```python
from build123d import *

# Parameters (mm, degrees)
SKETCH1_W           = 96
SKETCH1_H           = 68
BOSS_EXTRUDE1_DEPTH = 5
SKETCH2_R           = 1.65
SKETCH2_R_2         = 1.6
SKETCH2_R_3         = 7.5
CUT_EXTRUDE1_DEPTH  = 60.033888573


with BuildPart() as part:
    # Sketch1 → Boss-Extrude1 (new body)
    with BuildSketch(Plane(origin=(0, 0, 0), x_dir=(1, 0, 0), z_dir=(0, 1, 0))):
        Rectangle(SKETCH1_W, SKETCH1_H)
    extrude(amount=BOSS_EXTRUDE1_DEPTH)

    # Sketch2 → Cut-Extrude1 (cut, through all)
    with BuildSketch(Plane(origin=(0, 5, 0), x_dir=(1, 0, 0), z_dir=(0, 1, 0))):
        with Locations(Location((-43, 14, 0), (0, 0, 270))):
            Circle(SKETCH2_R)
        with Locations(Location((43, 14, 0), (0, 0, 270))):
            Circle(SKETCH2_R)
        with Locations(Location((43, -14, 0), (0, 0, 270))):
            Circle(SKETCH2_R)
        with Locations(Location((-43, -14, 0), (0, 0, 270))):
            Circle(SKETCH2_R)
        with Locations(Location((-11, 8, 0), (0, 0, 270))):
            Circle(SKETCH2_R_2)
        with Locations(Location((33, 8, 0), (0, 0, 270))):
            Circle(SKETCH2_R_2)
        with Locations(Location((33, -17, 0), (0, 0, 270))):
            Circle(SKETCH2_R_2)
        with Locations(Location((-11, -17, 0), (0, 0, 270))):
            Circle(SKETCH2_R_2)
        with Locations(Location((11, -3, 0), (0, 0, 270))):
            Circle(SKETCH2_R_3)
    extrude(amount=-CUT_EXTRUDE1_DEPTH, mode=Mode.SUBTRACT)


solid = part.part
```
The listing builds one solid part. Answer for the finished solid, in the listing's coordinates (mm). Give positions to 0.01 mm unless a question says otherwise; leave off trailing zeros. Order: outer loops, then holes, each group sorted by start corner. A loop starts at its lowest first (then second) coordinate and runs counter-clockwise, first axis right, second up. Notation, with made-up numbers: (29, 49.25) -> (65, 49.25) arc R33 cw to (65, 85.25) -> close; hole circle Ø7 at (81, 5). An arc over 180 degrees is marked (long way). Answer as a JSON object with one key per item and string values. Group by question number.
Item 1: The part is cut by section D-D on y = 3.5. Give the number of separate pieces and of enclosed holes in the cut face, and give its area (3 significant figures).
Item 2: The part is cut by section B-B on z = -14. Write down the section's boundary in (x, y).
Item 3: Consider L1, parallel to X at y = 3.5, z = -8; L2, parallel to X at y = 2, z = 14; L3, parallel to Z at x = -42, y = 2.5. Determine where each line is inside the solid, lowest interval first. Write a range as from..to.
Item 4: The part is cut by section C-C on x = 11. Write down the section's boundary in (y, z), and give its area (3 significant figures).
Item 5: The part is cut by section A-A on x = 43. Write down the section's boundary in (y, z), and give its area (3 significant figures).
Item 6: Determine the mould class of faces 1 (the cylindrical face through (32.03, 2.54, 15.73)), 2 (the flat face through (-1, 5, 0)), 3 (the flat face through (-1, 2, -34)) for opening direction Z: pulls with the +Z half, pulls with the -Z half, needs draft (parallel to the pull), parting line crosses it, or undercut.
Result set:
{
 "1": {"separate pieces": "1", "enclosed holes": "9", "area": "6,280 mm²"},
 "2": {"outline": "(-48, 0) -> (-44.65, 0) -> (-44.65, 5) -> (-48, 5) -> close; (-41.35, 0) -> (41.35, 0) -> (41.35, 5) -> (-41.35, 5) -> close; (44.65, 0) -> (48, 0) -> (48, 5) -> (44.65, 5) -> close"},
 "3": {"L1": "-48..-12.6, -9.4..31.4, 34.6..48", "L2": "-48..-44.65, -41.35..41.35, 44.65..48", "L3": "-34..-15.31, -12.69..12.69, 15.31..34"},
 "4": {"outline": "(0, -34) -> (5, -34) -> (5, -4.5) -> (0, -4.5) -> close; (0, 10.5) -> (5, 10.5) -> (5, 34) -> (0, 34) -> close", "area": "265 mm²"},
 "5": {"outline": "(0, -34) -> (5, -34) -> (5, -15.65) -> (0, -15.65) -> close; (0, -12.35) -> (5, -12.35) -> (5, 12.35) -> (0, 12.35) -> close; (0, 15.65) -> (5, 15.65) -> (5, 34) -> (0, 34) -> close", "area": "307 mm²"},
 "6": {"face 1": "undercut", "face 2": "needs draft", "face 3": "pulls with the -Z half"}
}
